Check sheet for the modelled part. Datum: model origin and axes. Units: mm. Coordinates: 2 decimals unless noted, no trailing zeros. Write each loop counter-clockwise with the first axis right and the second up, starting at its lowest first coordinate (ties: lowest second). Pieces come first, ordered by that corner, then holes. Notation, with made-up numbers: (6.25, 88.5) -> (50.25, 88.5) arc R15 ccw to (50.25, 95.5) -> close; hole circle Ø4 at (-36, 58.5). An arc over 180 degrees is marked (long way). One line per item, written item: value. Start each with the question number.
1) Sectioned sample at A-A on x = -136. Enter the section's corners in (y, z), plus the area to 3 significant figures.
2) Gauge pin test, flat end, axial feed: P1, Ø2, axis at x = -135.84, y = -58.9, coming from the -Z side. Record the tip position at first contact, or that the pin passes through.
3) Scan lines: line 1 along X through (y, z) = (-67.5, 0.1); line 2 along X through (y, z) = (-56, 0.15); line 3 along Y through (x, z) = (-137, 0.15). Record each from-to range of solid material in increasing order. Write a range as [from, to].
Autodesk Inventor part; units mm, degrees
ref_plane "YZ Plane" through (0, 0, 0) normal (1, 0, 0) x (0, 1, 0)
ref_plane "XZ Plane" through (0, 0, 0) normal (0, 1, 0) x (-1, 0, 0)
ref_plane "XY Plane" through (0, 0, 0) normal (0, 0, 1) x (1, 0, 0)
sketch "Sketch1" plane through (0, 0, 0) normal (0, 0, 1) x (1, 0, 0)
  line L0 (-139.8225, -42.851) -> (-139.8018, -82.2454)
  arc A0 (-138.8232, -41.8607) -> (-139.8225, -42.851) centre (-138.8223, -42.8609) ccw
  line L1 (-116.3009, -41.8403) -> (-138.8232, -41.8607)
  arc A1 (-115.3058, -42.8403) -> (-116.3009, -41.8403) centre (-116.306, -42.8405) ccw
  line L2 (-115.2978, -81.8628) -> (-115.3058, -42.8403)
  arc A2 (-116.299, -82.8549) -> (-115.2978, -81.8628) centre (-116.2978, -81.8549) ccw
  arc A3 (-139.8018, -82.2454) -> (-139.3074, -83.1072) centre (-138.8025, -82.2449) ccw
  line L3 (-116.0766, -82.8302) -> (-139.5966, -82.8514)
  circle A4 centre (-131.3626, -67.5261) radius 1.1
  circle A5 centre (-135.8392, -58.9026) radius 1.1
  point P0 (0, 0)
  dimension "d0" = 40.99
extrude "Extrusion1" add sketch "Sketch1" along normal blind 0.2
properties part number "Side Stiffener"
Answers:
1. outline: (-82.85, 0) -> (-59.99, 0) -> (-59.99, 0.2) -> (-82.85, 0.2) -> close; (-57.81, 0) -> (-41.86, 0) -> (-41.86, 0.2) -> (-57.81, 0.2) -> close
1. area: 7.76 mm2
2. P1: passes through
3. line 1: x = [-139.81, -132.46], [-130.26, -115.3]
3. line 2: x = [-139.82, -115.3]
3. line 3: y = [-82.85, -41.86]
